```python
from build123d import *

# Parameters (mm, degrees)
Y_KSEKLIK_EKSTR_ZYON1_DEPTH = 3
Y_KSEKLIK_EKSTR_ZYON2_DEPTH = 1.5
RADYUS1_R                   = 1
IZIM5_R                     = 1.6
KES_EKSTR_ZYON1_DEPTH       = 5
IZIM6_R                     = 3.75
KES_EKSTR_ZYON2_DEPTH       = 2


with BuildPart() as part:
    # Çizim1 → Yükseklik-Ekstrüzyon1 (new body)
    with BuildSketch(Plane.XY):
        with BuildLine():
            Line((-29.5, -26), (29.5, -26))
            ThreePointArc((29.5, -26), (36.571067812, -23.071067812), (39.5, -16))
            Line((39.5, -16), (39.5, 16))
            ThreePointArc((39.5, 16), (36.571067812, 23.071067812), (29.5, 26))
            Line((29.5, 26), (-29.5, 26))
            ThreePointArc((-29.5, 26), (-36.571067812, 23.071067812), (-39.5, 16))
            Line((-39.5, 16), (-39.5, -16))
            ThreePointArc((-39.5, -16), (-36.571067812, -23.071067812), (-29.5, -26))
        make_face()
    extrude(amount=Y_KSEKLIK_EKSTR_ZYON1_DEPTH)

    # Çizim4 → Yükseklik-Ekstrüzyon2 (add)
    with BuildSketch(Plane(origin=(0, 0, 0), x_dir=(-1, 0, 0), z_dir=(0, 0, -1))):
        with BuildLine():
            Line((-35.35, 16), (-35.35, -16))
            ThreePointArc((-35.35, -16), (-33.63657467, -20.13657467), (-29.5, -21.85))
            Line((-29.5, -21.85), (29.5, -21.85))
            ThreePointArc((29.5, -21.85), (33.63657467, -20.13657467), (35.35, -16))
            Line((35.35, -16), (35.35, 16))
            ThreePointArc((35.35, 16), (33.63657467, 20.13657467), (29.5, 21.85))
            Line((29.5, 21.85), (-29.5, 21.85))
            ThreePointArc((-29.5, 21.85), (-33.63657467, 20.13657467), (-35.35, 16))
        make_face()
    extrude(amount=Y_KSEKLIK_EKSTR_ZYON2_DEPTH)

    # Radyus1
    radyus1_edges = [part.edges().sort_by_distance(p)[0] for p in [
        (36.571067812, 23.071067812, 3),
        (0, 26, 3),
        (-36.571067812, 23.071067812, 3),
        (-39.5, 0, 3),
        (-36.571067812, -23.071067812, 3),
        (0, -26, 3),
        (36.571067812, -23.071067812, 3),
        (39.5, 0, 3),
    ]]
    fillet(radyus1_edges, radius=RADYUS1_R)

    # Çizim5 → Kes-Ekstrüzyon1 (cut)
    with BuildSketch(Plane.XY.offset(3)):
        with Locations((29.879306909, -18.598843149)):
            Circle(IZIM5_R)
        with Locations((-29.879306909, -18.598843149)):
            Circle(IZIM5_R)
        with Locations((-29.879306909, 18.598843149)):
            Circle(IZIM5_R)
        with Locations((29.879306909, 18.598843149)):
            Circle(IZIM5_R)
    extrude(amount=-KES_EKSTR_ZYON1_DEPTH, mode=Mode.SUBTRACT)

    # Çizim6 → Kes-Ekstrüzyon2 (cut)
    with BuildSketch(Plane.XY.offset(3)):
        with Locations((29.879306909, -18.598843149)):
            Circle(IZIM6_R)
        with Locations((-29.879306909, -18.598843149)):
            Circle(IZIM6_R)
        with Locations((-29.879306909, 18.598843149)):
            Circle(IZIM6_R)
        with Locations((29.879306909, 18.598843149)):
            Circle(IZIM6_R)
    extrude(amount=-KES_EKSTR_ZYON2_DEPTH, mode=Mode.SUBTRACT)


solid = part.part
```
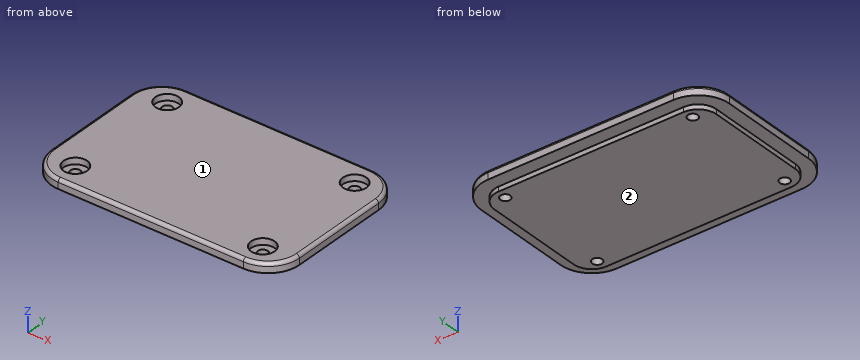
Can you work these out from the model? Positions are in its coordinate system, mm. Face numbers are marked on the shaded views. Coordinates: 2 decimals unless noted, no trailing zeros. Loops run counter-clockwise (first coordinate to the right, second up) from the corner with the lowest first, then second, coordinate; pieces in that order, holes last.
1) Thinking about a two-plate mould opening in Z: for the marked faces 1 and 2, which applies, pulls with the +Z half, pulls with the -Z half, needs draft (parallel to the pull), parting line crosses it, or undercut?
2) For pin 1 (6 mm diameter, centred on x = -29.88, y = -18.6, fed in from +Z); pin 2 (0.8 mm diameter, centred on x = -10.5, z = -0.5, fed in from +Y); pin 3 (1.6 mm diameter, centred on y = 0, z = -1, fed in from +X), each with a flat end and sliding along its axis, tell me the tip position at first contact or that it passes through.
3) Imagine slicing it at C-C on z = -0.7. List the corners of the cut face in (x, y) for me.
4) I need wall thicknesses on probe 1 along Y at (x, z) = (-30.5, 2.25); probe 2 along Z at (x, y) = (26, -22.5); probe 3 along X at (y, z) = (2, -0.35). Which ranges of each line are inside material? Lowest first, please.
5) Imagine slicing it at B-B on x = 13. List the corners of the cut face in (y, z) for me, plus the area to 3 significant figures.
6) Imagine slicing it at A-A on y = -1.5. List the corners of the cut face in (x, z) for me.
Completed:
1. face 1: pulls with the +Z half
1. face 2: pulls with the -Z half
2. pin 1: stops at z = 1
2. pin 2: stops at y = 21.85
2. pin 3: stops at x = 35.35
3. outline: (-35.35, -16) arc R5.85 ccw to (-29.5, -21.85) - (29.5, -21.85) arc R5.85 ccw to (35.35, -16) - (35.35, 16) arc R5.85 ccw to (29.5, 21.85) - (-29.5, 21.85) arc R5.85 ccw to (-35.35, 16) - close; hole circle Ø3.2 at (-29.88, -18.6); hole circle Ø3.2 at (-29.88, 18.6); hole circle Ø3.2 at (29.88, -18.6); hole circle Ø3.2 at (29.88, 18.6)
4. probe 1: y = -25.92 to -22.3, -14.9 to 14.9, 22.3 to 25.92
4. probe 2: z = 0 to 3
4. probe 3: x = -35.35 to 35.35
5. outline: (-26, 0) - (-21.85, 0) - (-21.85, -1.5) - (21.85, -1.5) - (21.85, 0) - (26, 0) - (26, 2) arc R1 ccw to (25, 3) - (-25, 3) arc R1 ccw to (-26, 2) - close
5. area: 221 mm2
6. outline: (-39.5, 0) - (-35.35, 0) - (-35.35, -1.5) - (35.35, -1.5) - (35.35, 0) - (39.5, 0) - (39.5, 2) arc R1 ccw to (38.5, 3) - (-38.5, 3) arc R1 ccw to (-39.5, 2) - close
